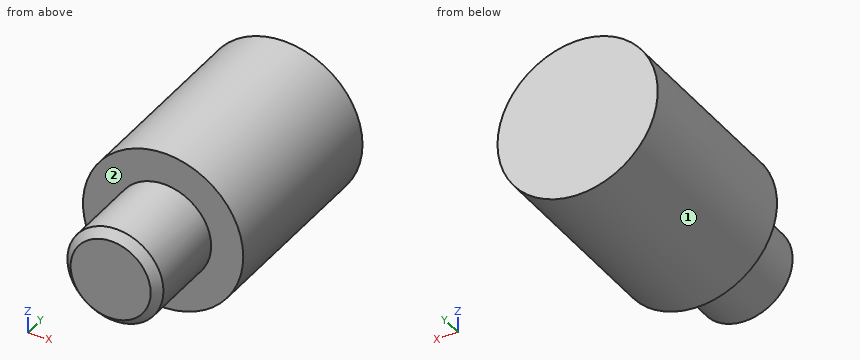
```python
from build123d import *

# Parameters (mm, degrees)
F0_R     = 10.01
F1_DEPTH = 25
F2_R     = 6
F3_DEPTH = 11
F4_SIZE2 = 1
F4_SIZE  = 1


with BuildPart() as f1:
    # F0 (on Front) → F1 (new body)
    with BuildSketch(Plane.XZ):
        Circle(F0_R)
    extrude(amount=F1_DEPTH)

    # F2 (on face) → F3 (join)
    with BuildSketch(Plane.XZ.offset(25)):
        Circle(F2_R)
    extrude(amount=F3_DEPTH)

    # F4
    f4_edges = [f1.edges().sort_by_distance(p)[0] for p in [
        (-6, -36, 0),
    ]]
    chamfer(f4_edges, length=F4_SIZE, length2=F4_SIZE2)


solid = f1.part
```
Geometry: final body of the model. Coordinates: model frame, mm. Face numbers are marked on the shaded views. A direction names the side the tool comes from. Round coordinates to 2 decimals unless told otherwise and drop trailing zeros. Write each loop counter-clockwise with the first axis right and the second up, starting at its lowest first coordinate (ties: lowest second). Pieces come first, ordered by that corner, then holes. Notation, with made-up numbers: M 77.5,63.5 L 95.5,63.5 A15 cw 95.5,82.5 Z; hole C -15,-13 d11. An arc over 180 degrees is marked long. Answer in a Markdown table with one row per item. Add a question column.
(1) Reachability of the marked faces 1 and 2 from +Z, -Z, +X, -X, +Y, -Y: full face, straight path, thin tool, end or side. Return the list, or none.
(2) Cut plane B-B, the plane z = 0. Return the cut outline in (x, y).
(3) Contact query for flat-ended pins moving along their axis: pin 1 (8 mm diameter, centred on x = 6, y = -26.5, fed in from +Z); pin 2 (3 mm diameter, centred on x = 5, y = -25, fed in from -Z); pin 3 (2 mm diameter, centred on x = -7, y = -7.5, fed in from +Z). Output: stop coordinate, or through.
(4) Cut plane C-C, the plane y = -12. Return the cut outline in (x, z).
(5) Cut plane A-A, the plane x = 0. Return the cut outline in (y, z), then the cut area to 4 significant figures.
(6) Cut plane D-D, the plane z = 8. Return the cut outline in (x, y).
(7) Ray query, L1, parallel to Y at x = -8.25, z = -2; L2, parallel to Z at x = 5, y = -29; L3, parallel to Z at x = 3.25, y = -33.5. Return the intervals inside material, ascending.
Established:
| question | item | result |
|---|---|---|
| 1 | face 1 | +Y, -Y |
| 1 | face 2 | -Y |
| 2 | outline | M -10.01,-25 L -6,-25 L -6,-35 L -5,-36 L 5,-36 L 6,-35 L 6,-25 L 10.01,-25 L 10.01,0 L -10.01,0 Z |
| 3 | pin 1 | z = 9.74 |
| 3 | pin 2 | z = -9.38 |
| 3 | pin 3 | z = 8.01 |
| 4 | outline | C 0,0 d20.02 |
| 5 | outline | M -36,-5 L -35,-6 L -25,-6 L -25,-10.01 L 0,-10.01 L 0,10.01 L -25,10.01 L -25,6 L -35,6 L -36,5 Z |
| 5 | area | 631.5 mm² |
| 6 | outline | M -6.02,-25 L 6.02,-25 L 6.02,0 L -6.02,0 Z |
| 7 | L1 | -25 to 0 |
| 7 | L2 | -3.32 to 3.32 |
| 7 | L3 | -5.04 to 5.04 |
